from build123d import *

# Parameters (mm, degrees)
SKETCH1_R               = 1.5
BOSS_EXTRUDE1_DEPTH     = 8
SKETCH2_R               = 2.75
BOSS_EXTRUDE2_DEPTH     = 2
CHAMFER1_SIZE           = 0.3
CUT_EXTRUDE1_DEPTH      = 9.895223437
CUT_EXTRUDE1_DEPTH_BACK = 9.895223437
SKETCH3_W               = 0.8
SKETCH3_H               = 1.7


with BuildPart() as part:
    # Sketch1 → Boss-Extrude1 (new body)
    with BuildSketch(Plane.XY):
        Circle(SKETCH1_R)
    extrude(amount=-BOSS_EXTRUDE1_DEPTH)

    # Sketch2 → Boss-Extrude2 (add)
    with BuildSketch(Plane.XY):
        Circle(SKETCH2_R)
    extrude(amount=BOSS_EXTRUDE2_DEPTH)

    # Chamfer1
    chamfer1_edges = [part.edges().sort_by_distance(p)[0] for p in [
        (-1.5, 0, -8),
        (-2.75, 0, 2),
    ]]
    chamfer(chamfer1_edges, length=CHAMFER1_SIZE)

    # Sketch3 → Cut-Extrude1 (cut, two sides: drawn at the far end of the back side and taken through both)
    with BuildSketch(Plane(origin=(0, 0, 0), x_dir=(1, 0, 0), z_dir=(0, 1, 0)).offset(-CUT_EXTRUDE1_DEPTH_BACK)):
        with Locations((0, -1.982738086)):
            Rectangle(SKETCH3_W, SKETCH3_H)
    extrude(amount=CUT_EXTRUDE1_DEPTH + CUT_EXTRUDE1_DEPTH_BACK, mode=Mode.SUBTRACT)


solid = part.part
Verification items for the finished model (mm, model axes). A direction names the side the tool comes from. Round coordinates to 2 decimals unless told otherwise and drop trailing zeros. Loops run counter-clockwise (first coordinate to the right, second up) from the corner with the lowest first, then second, coordinate; pieces in that order, holes last. Notation, with made-up numbers: (-5.5, -7) - (34.5, -7) arc R24 ccw to (34.5, 7) - close; hole circle Ø4 at (27, -27.5). An arc over 180 degrees is marked (long way). Use one line per item in the form item = value.
1. Section check A-A on y = 0. Record the cut outline in (x, z).
A:
outline = (-2.75, 0) - (-1.5, 0) - (-1.5, -7.7) - (-1.2, -8) - (1.2, -8) - (1.5, -7.7) - (1.5, 0) - (2.75, 0) - (2.75, 1.7) - (2.45, 2) - (0.4, 2) - (0.4, 1.13) - (-0.4, 1.13) - (-0.4, 2) - (-2.45, 2) - (-2.75, 1.7) - close
2. Section check C-C on z = -2.5. Record the cut outline in (x, y), and give its area (3 significant figures).
A:
outline = circle Ø3 at (0, 0)
area = 7.07 mm²
3. Section check D-D on z = 1. Record the cut outline in (x, y).
A:
outline = circle Ø5.5 at (0, 0)
4. Gauge pin test, flat ends, axial feed: pin 1 Ø0.6 at (x, y) = (0, -1) entering from +Z; pin 2 Ø2 at (y, z) = (1.5, -4) entering from -X; pin 3 Ø1 at (x, y) = (2, -1) entering from -Z. Record the tip position at first contact, or that the pin passes through.
A:
pin_1 = 1.13
pin_2 = -1.41
pin_3 = 0
5. Section check B-B on x = 0. Record the cut outline in (y, z), and give its area (3 significant figures).
A:
outline = (-2.75, 0) - (-1.5, 0) - (-1.5, -7.7) - (-1.2, -8) - (1.2, -8) - (1.5, -7.7) - (1.5, 0) - (2.75, 0) - (2.75, 1.13) - (-2.75, 1.13) - close
area = 30.1 mm²
6. Scan lines: probe 1 along Z at (x, y) = (0.2, -2.35); probe 2 along Y at (x, z) = (-0.1, -6); probe 3 along Z at (x, y) = (-0.35, -0.6). Record each from-to range of solid material in increasing order.
A:
probe_1 = 0 to 1.13
probe_2 = -1.5 to 1.5
probe_3 = -8 to 1.13
7. Access from +Z, -Z, +X, -X, +Y, -Y to the whole of each face (thin tool, end or side, straight path). Record for faces 1 (the flat face through (0, 0, 1.133)), 2 (the flat face through (1.2, -1.2, 0)), 3 (the flat face through (-1, 0, 2)).
A:
face_1 = +Z, +Y, -Y
face_2 = -Z
face_3 = +Z, +X, -X, +Y, -Y
8. Draft check along X on faces 4 (the flat face through (-0.4, 0, 1.6)), 5 (the cylindrical face through (-1.5, 0.07, -3.8)), 6 (the flat face through (0.4, 0, 1.6)), 7 (the flat face through (1, 0, 2)). Enter one of: pulls with the +X half, pulls with the -X half, needs draft (parallel to the pull), parting line crosses it, or undercut.
A:
face_4 = undercut
face_5 = parting line crosses it
face_6 = undercut
face_7 = needs draft
